Can you work these out from the model? Positions are in its coordinate system, mm. Face numbers are marked on the shaded views. Give positions to 0.01 mm unless a question says otherwise; leave off trailing zeros. Loops run counter-clockwise (first coordinate to the right, second up) from the corner with the lowest first, then second, coordinate; pieces in that order, holes last. Notation, with made-up numbers: (4.5, 22.25) - (60.5, 22.25) arc R28 cw to (60.5, 48.25) - close; hole circle Ø9 at (27, 52.5). An arc over 180 degrees is marked (long way). Write item = value, one per line.
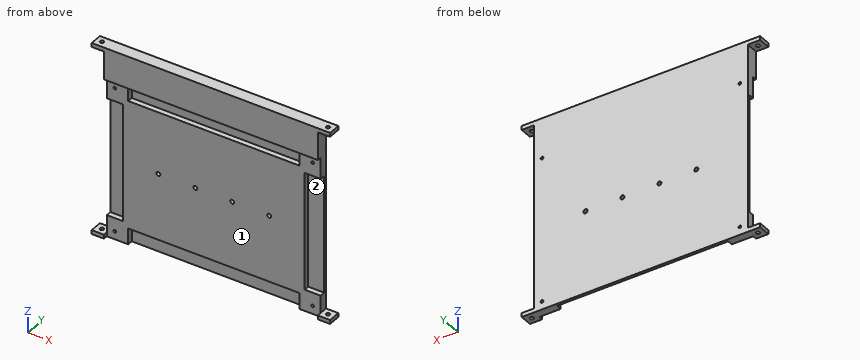
from build123d import *

# Parameters (mm, degrees)
SKETCH_1_W          = 80
SKETCH_1_H          = 3
EXTRUDE_1_DEPTH     = 60
SKETCH_4_R          = 0.5
CUT_EXTRUDE_1_DEPTH = 73.173402303
SKETCH_5_W          = 64
SKETCH_5_H          = 6
SKETCH_5_W_2        = 6
SKETCH_5_H_2        = 44
CUT_EXTRUDE_4_DEPTH = 2
EXTRUDE_START       = -60
SKETCH_6_R          = 0.7
EXTRUDE_2_DEPTH     = 1.5
EXTRUDE_3_DEPTH     = 12
EXTRUDE_START_2     = 10.5
SKETCH_6_4_R        = 0.7
EXTRUDE_4_DEPTH     = 1.5
SKETCH_7_R          = 0.75
CUT_EXTRUDE_5_DEPTH = 85.819337418


with BuildPart() as part:
    # 草图1 → 凸台-拉伸1 (new body)
    with BuildSketch(Plane.XY):
        Rectangle(SKETCH_1_W, SKETCH_1_H)
    extrude(amount=EXTRUDE_1_DEPTH)

    # 草图4 → 切除-拉伸1 (cut, through all)
    with BuildSketch(Plane(origin=(0, 1.5, 0), x_dir=(1, 0, 0), z_dir=(0, 1, 0))):
        with Locations(Location((-37, -57, 0), (0, 0, 270))):
            Circle(SKETCH_4_R)
        with Locations(Location((37, -57, 0), (0, 0, 270))):
            Circle(SKETCH_4_R)
        with Locations(Location((-37, -3, 0), (0, 0, 270))):
            Circle(SKETCH_4_R)
        with Locations(Location((37, -3, 0), (0, 0, 270))):
            Circle(SKETCH_4_R)
    extrude(amount=-CUT_EXTRUDE_1_DEPTH, mode=Mode.SUBTRACT)

    # 草图5 → 切除-拉伸4 (cut)
    with BuildSketch(Plane.XZ.offset(1.5)):
        with Locations((0, 57)):
            Rectangle(SKETCH_5_W, SKETCH_5_H)
        with Locations((37, 30)):
            Rectangle(SKETCH_5_W_2, SKETCH_5_H_2)
        with Locations((0, 3)):
            Rectangle(SKETCH_5_W, SKETCH_5_H)
        with Locations((-37, 30)):
            Rectangle(SKETCH_5_W_2, SKETCH_5_H_2)
    extrude(amount=-CUT_EXTRUDE_4_DEPTH, mode=Mode.SUBTRACT)

    # 草图6 → 凸台-拉伸2 (add)
    # profile 1 of 2: a face of its own
    with BuildSketch(Plane.XY.offset(60).offset(EXTRUDE_START)):
        Polygon((-40, -1.5), (-40, 1.5), (-44.6, 1.5), (-44.6, -3.1), (-40, -3.1), align=None)
        with Locations((-42.3, -0.8)):
            Circle(SKETCH_6_R, mode=Mode.SUBTRACT)
    # profile 2 of 2: a face of its own
    with BuildSketch(Plane.XY.offset(60).offset(EXTRUDE_START)):
        Polygon((44.6, 1.5), (40, 1.5), (40, -1.5), (40, -3.1), (44.6, -3.1), align=None)
        with Locations((42.3, -0.8)):
            Circle(SKETCH_6_R, mode=Mode.SUBTRACT)
    extrude(amount=EXTRUDE_2_DEPTH)

    # 草图6<3> → 凸台-拉伸3 (add)
    with BuildSketch(Plane.XY.offset(60)):
        Polygon((-32, -1.5), (-40, -1.5), (-40, -3.1), (40, -3.1), (40, -1.5), (32, -1.5), (32, 0.5), (-32, 0.5), align=None)
        Polygon((-40, -1.5), (-32, -1.5), (-32, 0.5), (32, 0.5), (32, -1.5), (40, -1.5), (40, 1.5), (-40, 1.5), align=None)
    extrude(amount=EXTRUDE_3_DEPTH)

    # 草图6<4> → 凸台-拉伸4 (add)
    # profile 1 of 2: a face of its own
    with BuildSketch(Plane.XY.offset(60).offset(EXTRUDE_START_2)):
        Polygon((-40, -1.5), (-40, 1.5), (-44.6, 1.5), (-44.6, -3.1), (-40, -3.1), align=None)
        with Locations((-42.3, -0.8)):
            Circle(SKETCH_6_4_R, mode=Mode.SUBTRACT)
    # profile 2 of 2: a face of its own
    with BuildSketch(Plane.XY.offset(60).offset(EXTRUDE_START_2)):
        Polygon((44.6, 1.5), (40, 1.5), (40, -1.5), (40, -3.1), (44.6, -3.1), align=None)
        with Locations((42.3, -0.8)):
            Circle(SKETCH_6_4_R, mode=Mode.SUBTRACT)
    extrude(amount=EXTRUDE_4_DEPTH)

    # 草图7 → 切除-拉伸5 (cut, through all)
    with BuildSketch(Plane(origin=(0, 1.5, 0), x_dir=(1, 0, 0), z_dir=(0, 1, 0))):
        with Locations(Location((20.7375, -30.8, 0), (0, 0, 270))):
            Circle(SKETCH_7_R)
        with Locations(Location((6.9125, -30.8, 0), (0, 0, 270))):
            Circle(SKETCH_7_R)
        with Locations(Location((-6.9125, -30.8, 0), (0, 0, 270))):
            Circle(SKETCH_7_R)
        with Locations(Location((-20.7375, -30.8, 0), (0, 0, 270))):
            Circle(SKETCH_7_R)
    extrude(amount=-CUT_EXTRUDE_5_DEPTH, mode=Mode.SUBTRACT)


solid = part.part
Q1. Imagine slicing it at C-C, the plane y = -0.8. Give the number of separate pieces and of enclosed holes in the cut face, then the cut area to 3 significant figures.
Output:
separate_pieces = 5
enclosed_holes = 9
area = 4,470 mm2
Q2. For pin 1 (6.5 mm diameter, centred on x = 36, z = 28.5, fed in from -Y); pin 2 (1.8 mm diameter, centred on x = -36.5, z = 36, fed in from -Y); pin 3 (1.1 mm diameter, centred on x = 42.3, y = -0.8, fed in from +Z) (3 decimals), each with a flat end and sliding along its axis, tell me the tip position at first contact or that it passes through.
Output:
pin_1 = -1.5
pin_2 = 0.5
pin_3 = through
Q3. Imagine slicing it at D-D, the plane x = 24. Write out the boundary of the cut face in (y, z), then the cut area to 3 significant figures.
Output:
outline = (-3.1, 60) - (0.5, 60) - (0.5, 54) - (-1.5, 54) - (-1.5, 6) - (0.5, 6) - (0.5, 0) - (1.5, 0) - (1.5, 72) - (-3.1, 72) - close
area = 211 mm2
Q4. Imagine slicing it at A-A, the plane x = 33. Write out the boundary of the cut face in (y, z).
Output:
outline = (-3.1, 60) - (-1.5, 60) - (-1.5, 0) - (1.5, 0) - (1.5, 72) - (-3.1, 72) - close
Q5. We'd pull the mould along Z, two halves only. Please class the marked faces 1 and 2: released by +Z, released by -Z, zero draft, split by the parting line, or undercut.
Output:
face_1 = zero draft
face_2 = undercut
Q6. I need wall thicknesses on L1, parallel to X at y = 0.2, z = 3; L2, parallel to X at y = -0.3, z = 30.8; L3, parallel to X at y = 0.85, z = 57. Which ranges of each line are inside material? Lowest first, please.
Output:
L1 = -40 to -37.5, -36.5 to -32, 32 to 36.5, 37.5 to 40
L2 = -34 to -21.49, -19.99 to -7.66, -6.16 to 6.16, 7.66 to 19.99, 21.49 to 34
L3 = -40 to -37.5, -36.5 to 36.5, 37.5 to 40
Q7. Imagine slicing it at B-B, the plane z = 55.5. Write out the boundary of the cut face in (x, y).
Output:
outline = (-40, -1.5) - (-32, -1.5) - (-32, 0.5) - (32, 0.5) - (32, -1.5) - (40, -1.5) - (40, 1.5) - (-40, 1.5) - close
